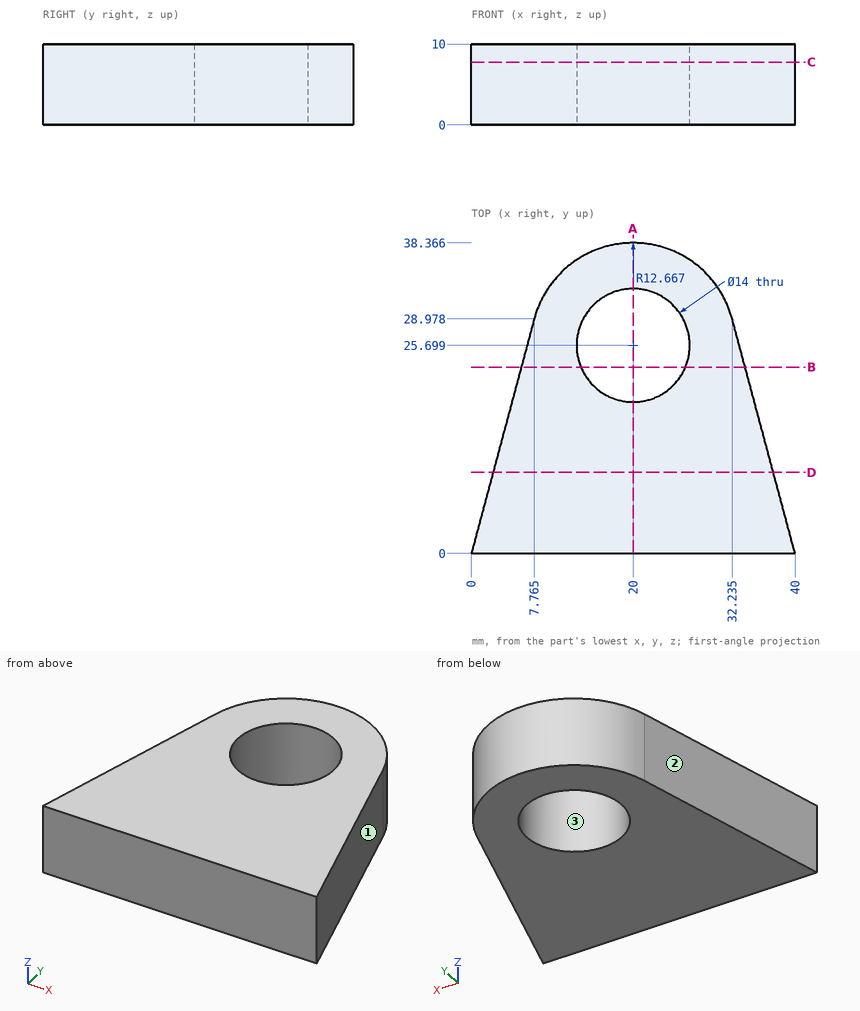
Check sheet for the drawn part. Datum: minimum x, y, z corner. Units: mm. Round coordinates to 2 decimals unless told otherwise and drop trailing zeros. Order: outer loops, then holes, each group sorted by start corner. A loop starts at its lowest first (then second) coordinate and runs counter-clockwise, first axis right, second up. Notation, with made-up numbers: (30, -9.5) -> (48, -9.5) arc R21 cw to (48, 5.5) -> close; hole circle Ø8 at (-12, 40). An arc over 180 degrees is marked (long way). Put each result on its own line as item: value.
1) Section check A-A (x = 20). Record the cut outline in (y, z).
Final values:
outline: (0, 0) -> (18.7, 0) -> (18.7, 10) -> (0, 10) -> close; (32.7, 0) -> (38.37, 0) -> (38.37, 10) -> (32.7, 10) -> close
2) Section check D-D (y = 10). Record the cut outline in (x, z).
Final values:
outline: (2.68, 0) -> (37.32, 0) -> (37.32, 10) -> (2.68, 10) -> close
3) Material ranges on line 1 (X direction, y = 28, z = 8.25); line 2 (X direction, y = 25, z = 1.75) (1 decimal); line 3 (Y direction, x = 24.5, z = 7.75), recorded low to high.
Final values:
line 1: x = 7.5 to 13.39, 26.61 to 32.5
line 2: x = 6.7 to 13, 27 to 33.3
line 3: y = 0 to 20.34, 31.06 to 37.54
4) Depth check by flat-ended pin: pin 1 (5 mm diameter, centred on x = 33.5, z = 7.5, fed in from +Y); pin 2 (1 mm diameter, centred on x = 33, y = 25, fed in from -Z); pin 3 (4 mm diameter, centred on y = 12.5, z = 8, fed in from +X); pin 4 (3 mm diameter, centred on y = 30.5, z = 8.5, fed in from -X). Enter the tip coordinate at first touch or a pass-through.
Final values:
pin 1: stops at y = 31.98
pin 2: stops at z = 0
pin 3: stops at x = 37.19
pin 4: stops at x = 7.77
5) Section check B-B (y = 23). Record the cut outline in (x, z).
Final values:
outline: (6.16, 0) -> (13.54, 0) -> (13.54, 10) -> (6.16, 10) -> close; (26.46, 0) -> (33.84, 0) -> (33.84, 10) -> (26.46, 10) -> close
6) Section check C-C (z = 7.75). Record the cut outline in (x, y) (1 decimal), then the cut area to 3 significant figures.
Final values:
outline: (0, 0) -> (40, 0) -> (32.2, 29) arc R12.7 ccw to (7.8, 29) -> close; hole circle Ø14 at (20, 25.7)
area: 950 mm^2
7) Mould release check, pull along X, two halves, no side actions. Record for the marked faces 1, 2 and 3: +X half, -X half, draft (parallel to the pull), parting line (faces both ways), or undercut.
Final values:
face 1: +X half
face 2: -X half
face 3: undercut
